Can you work these out from the model? Positions are in its coordinate system, mm. A direction names the side the tool comes from. Give positions to 0.01 mm unless a question says otherwise; leave off trailing zeros. Write each loop counter-clockwise with the first axis right and the second up, starting at its lowest first coordinate (ties: lowest second). Pieces come first, ordered by that corner, then holes. Notation, with made-up numbers: (0, 75.5) -> (31, 75.5) arc R26 cw to (31, 98.5) -> close; hole circle Ø9 at (71, -38). An arc over 180 degrees is marked (long way). Answer as CSV lines item,"result". Start each with the question number.
1. If we section it at B-B on z = 1174: Write out the boundary of the cut face in (x, y), plus the area to 3 significant figures.
2. On a 3-axis mill with a long thin cutter (end or side, diameter ignored), from which of +Z, -Z, +X, -X, +Y, -Y can I reach the whole of each face in a straight line? I mean faces 4 (the face through (-840, 25, 25)), 5 (the face through (-25, 25, 0)), 6 (the face through (-451, 300, 635)). Say none if no direction works.
3. If we section it at C-C on y = 197: Write out the boundary of the cut face in (x, z).
4. If we mould it in two halves opening along Z, with no side actions, what happens to faces 1 (the face through (-451, 148, 1920)), 2 (the face through (-865, 50, 25)), 3 (the face through (-865, 315, 0))? For each: pulls with the +Z half, pulls with the -Z half, needs draft (parallel to the pull), parting line crosses it, or undercut.
5. I need wall thicknesses on line 1 (X direction, y = 196.5, z = 997); line 2 (Y direction, x = -68, z = 231); line 3 (Z direction, x = -617, y = 300.5). Which ranges of each line are inside material? Lowest first, please. Write a range as [from, to].
6. I'm going to push a flat-ended pin straight in: P1, Ø6, axis at x = -322.5, z = 898, coming from the -Y side. Where does the tip first touch, or does it pass through?
7. If we section it at D-D on x = -454.5: Write out the boundary of the cut face in (y, z).
8. If we section it at A-A on y = 319: Write out the boundary of the cut face in (x, z), plus the area to 3 significant figures.
```python
from build123d import *

# Parameters (mm, degrees)
F0_W     = 890
F0_H     = 340
F1_DEPTH = 1970
F2_W     = 790
F2_H     = 50
F3_DEPTH = 350
F2_H_2   = 380
F2_H_3   = 270
F4_DEPTH = 300
F5_W     = 240
F5_H     = 50
F6_DEPTH = 895


with BuildPart() as f1:
    # F0 (on Top) → F1 (new body)
    with BuildSketch(Plane.XY):
        with Locations((-445, 170)):
            Rectangle(F0_W, F0_H)
    extrude(amount=F1_DEPTH)

    # F2 (on face) → F3 (cut)
    with BuildSketch(Plane.XZ):
        with Locations((-445, 25)):
            Rectangle(F2_W, F2_H)
    extrude(amount=-F3_DEPTH, mode=Mode.SUBTRACT)

    # F2 (on face) → F4 (cut)
    with BuildSketch(Plane.XZ):
        with Locations((-445, 290)):
            Rectangle(F2_W, F2_H_2)
        with Locations((-445, 633)):
            Rectangle(F2_W, F2_H_3)
        with Locations((-445, 921)):
            Rectangle(F2_W, F2_H_3)
        with Locations((-445, 1209)):
            Rectangle(F2_W, F2_H_3)
        with Locations((-445, 1497)):
            Rectangle(F2_W, F2_H_3)
        with Locations((-445, 1785)):
            Rectangle(F2_W, F2_H_3)
    extrude(amount=-F4_DEPTH, mode=Mode.SUBTRACT)

    # F5 (on face) → F6 (cut)
    with BuildSketch(Plane(origin=(-890, 0, 0), x_dir=(0, -1, 0), z_dir=(-1, 0, 0))):
        with Locations((-170, 25)):
            Rectangle(F5_W, F5_H)
    extrude(amount=-F6_DEPTH, mode=Mode.SUBTRACT)


solid = f1.part
```
Computed values:
1,outline,"(-890, 0) -> (-840, 0) -> (-840, 300) -> (-50, 300) -> (-50, 0) -> (0, 0) -> (0, 340) -> (-890, 340) -> close"
1,area,"65,600 mm2"
2,face 4,"-Z, +Y, -Y"
2,face 5,"-Z, +X, -X, +Y, -Y"
2,face 6,"-Y"
3,outline,"(-890, 50) -> (0, 50) -> (0, 1970) -> (-890, 1970) -> close; hole (-840, 100) -> (-50, 100) -> (-50, 480) -> (-840, 480) -> close; hole (-840, 498) -> (-50, 498) -> (-50, 768) -> (-840, 768) -> close; hole (-840, 786) -> (-50, 786) -> (-50, 1056) -> (-840, 1056) -> close; hole (-840, 1074) -> (-50, 1074) -> (-50, 1344) -> (-840, 1344) -> close; hole (-840, 1362) -> (-50, 1362) -> (-50, 1632) -> (-840, 1632) -> close; hole (-840, 1650) -> (-50, 1650) -> (-50, 1920) -> (-840, 1920) -> close"
4,face 1,"undercut"
4,face 2,"needs draft"
4,face 3,"pulls with the -Z half"
5,line 1,"x = [-890, -840], [-50, 0]"
5,line 2,"y = [300, 340]"
5,line 3,"z = [50, 1970]"
6,P1,"stops at y = 300"
7,outline,"(0, 50) -> (340, 50) -> (340, 1970) -> (0, 1970) -> (0, 1920) -> (300, 1920) -> (300, 1650) -> (0, 1650) -> (0, 1632) -> (300, 1632) -> (300, 1362) -> (0, 1362) -> (0, 1344) -> (300, 1344) -> (300, 1074) -> (0, 1074) -> (0, 1056) -> (300, 1056) -> (300, 786) -> (0, 786) -> (0, 768) -> (300, 768) -> (300, 498) -> (0, 498) -> (0, 480) -> (300, 480) -> (300, 100) -> (0, 100) -> close"
8,outline,"(-890, 0) -> (-840, 0) -> (-840, 50) -> (-50, 50) -> (-50, 0) -> (0, 0) -> (0, 1970) -> (-890, 1970) -> close"
8,area,"1,710,000 mm2"
